The listing builds one solid part. Answer for the finished solid, in the listing's coordinates (mm). A direction names the side the tool comes from. Round coordinates to 2 decimals unless told otherwise and drop trailing zeros. Write each loop counter-clockwise with the first axis right and the second up, starting at its lowest first coordinate (ties: lowest second). Pieces come first, ordered by that corner, then holes.
(1) For faces 1 (the face through (58.247, -0.143, 19.084)), 2 (the face through (106.7, -0.07, 6.59)), determine the directions among +Z, -Z, +X, -X, +Y, -Y from which every point of the face is accessible in a straight line to the end or side of a thin tool.
(2) The mould has two halves that part along X. Classify faces 3 (the face through (103.6, -1.4, 13)), 4 (the face through (87, 6, 0)), 5 (the face through (53.6, -1.4, 13)), 6 (the face through (41.79, -3.92, 9.55)): +X half, -X half, draft (parallel to the pull), parting line (faces both ways), or undercut.
(3) A cutting plane is placed at D-D, the plane x = 55. Give the vertices of the cut face in (y, z), and give its area (3 significant figures).
(4) A cutting plane is placed at A-A, the plane x = 105. Give the vertices of the cut face in (y, z).
(5) A cutting plane is placed at C-C, the plane z = 7.75. Give the vertices of the cut face in (x, y), and give its area (3 significant figures).
(6) Each of these flat-tipped pins is pushed along its axis until it touches: pin 1 Ø8 at (x, z) = (115.5, 16) entering from +Y; pin 2 Ø2 at (x, y) = (56, 1) entering from +Z; pin 3 Ø6 at (x, z) = (76.5, 11.5) entering from -Y; pin 4 Ø2 at (x, y) = (55, 0) entering from +Z. Where does it stop, or does it pass through?
(7) A cutting plane is placed at B-B, the plane y = 0. Give the vertices of the cut face in (x, z), and give its area (3 significant figures).
(8) Find the intervals of material crossed by probe 1 along X at (y, z) = (-2, 21); probe 2 along X at (y, z) = (0, 21.75); probe 3 along Y at (x, z) = (57.5, 15), in increasing order.
Autodesk Inventor part; units mm, degrees
ref_plane "Plan de construction1" through (115, -25, 25) normal (0, 0, -1) x (-1, 0, 0)
ref_plane "Plan YZ" through (0, 0, 0) normal (1, 0, 0) x (0, 1, 0)
ref_plane "Plan XZ" through (0, 0, 0) normal (0, 1, 0) x (-1, 0, 0)
sketch "Esquisse1" plane through (0, 0, 0) normal (0, 0, 1) x (1, 0, 0)
  arc A0 (25, 25) -> (0, 0) centre (25, 0) ccw
  line L0 (25, 25) -> (115, 25)
  arc A1 (140, 0) -> (115, 25) centre (115, 0) ccw
  line L1 (0, 0) -> (132.1239, 0) construction
  line L2 (0, 0) -> (140, 0)
  dimension "d0" = 25
  dimension "d1" = 90
revolve "Révolution1" add sketch "Esquisse1" angle 180 about axis through (0, 0, 0) along (1, 0, 0)
sketch "Esquisse6" plane through (115, 25, 0) normal (0, 0, -1) x (-1, 0, 0)
  line L0 (36.6987, -50) -> (51.6987, -75.9808)
  line L1 (51.6987, -75.9808) -> (115, -39.4338)
  arc A0 (90, -50) -> (90, 0) centre (90, -25) ccw
  line L2 (90, 0) -> (0, 0)
  line L3 (115, -25) -> (-35.1202, -25) construction
  line L4 (0, -50) -> (90, -50)
  line L5 (108.7132, -8.4224) -> (36.6987, -50)
  line L6 (108.7132, -8.4224) -> (115, -8.4224)
  line L7 (115, -8.4224) -> (115, -39.4338)
  dimension "d17" = 30
  dimension "d18" = 30
extrude "Extrusion1" cut sketch "Esquisse6" against normal blind 25
ref_plane "Plan de construction1" through (115, -25, 25) normal (0, 0, -1) x (-1, 0, 0)
sketch "Esquisse7" plane through (115, -25, 25) normal (0, 0, -1) x (-1, 0, 0)
  circle A0 centre (10, 25) radius 1.7
  circle A1 centre (60, 25) radius 1.7
  line L0 (0, 50) -> (0, 0)
  line L1 (10, 25) -> (10, 0) construction
  line L2 (10, 25) -> (10, 50) construction
  line L3 (60, 25) -> (60, 0) construction
  line L4 (60, 25) -> (60, 50) construction
  line L5 (0, 50) -> (95.4771, 50) construction
  line L6 (0, 0) -> (90, 0) construction
  point P0 (115, 25)
  dimension "d7" = 10
  dimension "d8" = 50
  dimension "d9" = 3.4
  dimension "d10" = 3.4
extrude "Extrusion2" cut sketch "Esquisse7" along normal blind 25
sketch "Esquisse8" plane through (115, -25, 25) normal (0, 0, -1) x (-1, 0, 0)
  circle A0 centre (10, 25) radius 3.25
  circle A1 centre (60, 25) radius 3.25
  circle A2 centre (10, 25) radius 1.7
  circle A3 centre (60, 25) radius 1.7
  point P0 (115, 25)
  dimension "d13" = 6.5
  dimension "d14" = 6.5
extrude "Extrusion3" cut sketch "Esquisse8" along normal blind 12 contours A0 | A1 | A2 | A3
equation "\"d10\" = d9"
equation "\"d14\" = d13"
properties part number "P1704_003" material "."
Solutions:
1. face 1: +Z
1. face 2: +Z, -Z
2. face 3: undercut
2. face 4: draft
2. face 5: undercut
2. face 6: -X half
3. outline: (-11.55, 0) - (-1.7, 0) - (-1.7, 13) - (-3.25, 13) - (-3.25, 24.79) arc R25 ccw to (-11.55, 22.17) - close; (1.7, 0) - (25, 0) arc R25 ccw to (3.25, 24.79) - (3.25, 13) - (1.7, 13) - close
3. area: 647 mm2
4. outline: (-25, 0) - (-1.7, 0) - (-1.7, 13) - (-3.25, 13) - (-3.25, 24.79) arc R25 ccw to start; (1.7, 0) - (25, 0) arc R25 ccw to (3.25, 24.79) - (3.25, 13) - (1.7, 13) - close
5. outline: (7.38, 15.95) - (76.17, -23.77) - (115, -23.77) arc R23.77 ccw to (115, 23.77) - (25, 23.77) arc R23.77 ccw to start; hole circle Ø3.4 at (55, 0); hole circle Ø3.4 at (105, 0)
5. area: 4,580 mm2
6. pin 1: stops at y = 21.93
6. pin 2: stops at z = 13
6. pin 3: stops at y = -23.51
6. pin 4: passes through
7. outline: (35, 0) - (53.3, 0) - (53.3, 13) - (51.75, 13) - (51.75, 25) - (35, 25) - close; (56.7, 0) - (103.3, 0) - (103.3, 13) - (101.75, 13) - (101.75, 25) - (58.25, 25) - (58.25, 13) - (56.7, 13) - close; (106.7, 0) - (140, 0) arc R25 ccw to (115, 25) - (108.25, 25) - (108.25, 13) - (106.7, 13) - close
7. area: 2,250 mm2
8. probe 1: x = 38.46 to 52.44, 57.56 to 102.44, 107.56 to 128.42
8. probe 2: x = 35 to 51.75, 58.25 to 101.75, 108.25 to 127.33
8. probe 3: y = -12.99 to -2.08, 2.08 to 20
